Design review of the part built by this model. Coordinates are the model's own, in mm. A direction names the side the tool comes from. Round coordinates to 2 decimals unless told otherwise and drop trailing zeros. Loops run counter-clockwise (first coordinate to the right, second up) from the corner with the lowest first, then second, coordinate; pieces in that order, holes last. Notation, with made-up numbers: (6, 0) -> (56, 0) arc R25 ccw to (56, 16) -> close; hole circle Ø3 at (1.25, -16). An arc over 180 degrees is marked (long way). Answer as CSV lines item,"result". Start each with the question number.
(1) Draft analysis for pull direction Z (two halves, no side actions). For faces 1 (the face through (31, 0, -25.68)), 2 (the face through (31, -35.482, 0)), 3 (the face through (33.275, 0, 0)), state which applies: +Z half, -Z half, draft (parallel to the pull), parting line (faces both ways), or undercut.
(2) Take a section at A-A, the plane y = -19.5. Write out the cut boundary in (x, z).
(3) For P1, Ø19, axis at y = 0, z = 1, coming from the +X side, flat-tipped, find the tip position at first contact; note if it passes through.
(4) To check wall thickness, follow line 1 (Y direction, x = 33.5, z = -13.5); line 2 (Z direction, x = 35, y = 27); line 3 (X direction, y = -0.5, z = 14). State the ranges of each line that lie inside material, in increasing order. Write a range as from..to.
(5) Take a section at B-B, the plane z = 18. Write out the cut boundary in (x, y).
(6) Machinability: for faces 4 (the face through (30.534, -32.907, -23.176)), 5 (the face through (35, 0, 19.031)), which of the approach directions +Z, -Z, +X, -X, +Y, -Y give a long, thin tool a straight path to every point of the face, cutting with its end or side? Answer none if there is none.
from build123d import *

# Parameters (mm, degrees)
F0_W      = 70.9643363953
F0_H      = 51.3598918915
F1_DEPTH  = 76.2
F2_DEPTH  = 25.4
F3_DEPTH  = 40.3854846954
F4_DEPTH  = 25.4
F5_W      = 61.9144514203
F5_H      = 38.062274456
F6_DEPTH  = 2.54
F7_SIZE   = 5.08
F8_SIZE   = 5.08
F9_SIZE   = 5.08
F10_SIZE  = 5.08
F11_DEPTH = 25.4


with BuildPart() as f1:
    # F0 (on Right) → F1 (new body)
    with BuildSketch(Plane.YZ):
        Rectangle(F0_W, F0_H)
    extrude(amount=F1_DEPTH)

    # F2 (add): a face of the model
    f2_faces = [f1.faces().sort_by_distance(p)[0] for p in [
        (76.2, 0, 0),
    ]]
    extrude(f2_faces, amount=F2_DEPTH)

    # F3 (cut): a face of the model
    f3_faces = [f1.faces().sort_by_distance(p)[0] for p in [
        (101.6, 0, 0),
    ]]
    extrude(f3_faces, amount=-F3_DEPTH, mode=Mode.SUBTRACT)

    # F4 (cut): a face of the model
    f4_faces = [f1.faces().sort_by_distance(p)[0] for p in [
        (61.2145153046, 0, 0),
    ]]
    extrude(f4_faces, amount=-F4_DEPTH, mode=Mode.SUBTRACT)

    # F5 (on face) → F6 (cut)
    with BuildSketch(Plane.YZ.offset(35.8145153046)):
        Rectangle(F5_W, F5_H)
    extrude(amount=-F6_DEPTH, mode=Mode.SUBTRACT)

    # F7
    f7_edges = [f1.edges().sort_by_distance(p)[0] for p in [
        (17.907258, -35.482168, 25.679946),
    ]]
    chamfer(f7_edges, length=F7_SIZE)

    # F8
    f8_edges = [f1.edges().sort_by_distance(p)[0] for p in [
        (17.907258, -35.482168, -25.679946),
    ]]
    chamfer(f8_edges, length=F8_SIZE)

    # F9
    f9_edges = [f1.edges().sort_by_distance(p)[0] for p in [
        (17.907258, 35.482168, 25.679946),
    ]]
    chamfer(f9_edges, length=F9_SIZE)

    # F10
    f10_edges = [f1.edges().sort_by_distance(p)[0] for p in [
        (17.907258, 35.482168, -25.679946),
    ]]
    chamfer(f10_edges, length=F10_SIZE)

    # F11 (cut): a face of the model
    f11_faces = [f1.faces().sort_by_distance(p)[0] for p in [
        (0, 0, 0),
    ]]
    extrude(f11_faces, amount=-F11_DEPTH, mode=Mode.SUBTRACT)


solid = f1.part
The answers:
1,face 1,"-Z half"
1,face 2,"draft"
1,face 3,"undercut"
2,outline,"(25.4, -25.68) -> (35.81, -25.68) -> (35.81, -19.03) -> (33.27, -19.03) -> (33.27, 19.03) -> (35.81, 19.03) -> (35.81, 25.68) -> (25.4, 25.68) -> close"
3,P1,"x = 33.27"
4,line 1,"-35.48..-30.96, 30.96..35.48"
4,line 2,"-25.68..-19.03, 19.03..25.68"
4,line 3,"25.4..33.27"
5,outline,"(25.4, -35.48) -> (35.81, -35.48) -> (35.81, -30.96) -> (33.27, -30.96) -> (33.27, 30.96) -> (35.81, 30.96) -> (35.81, 35.48) -> (25.4, 35.48) -> close"
6,face 4,"-Z, +X, -X, -Y"
6,face 5,"+X"
